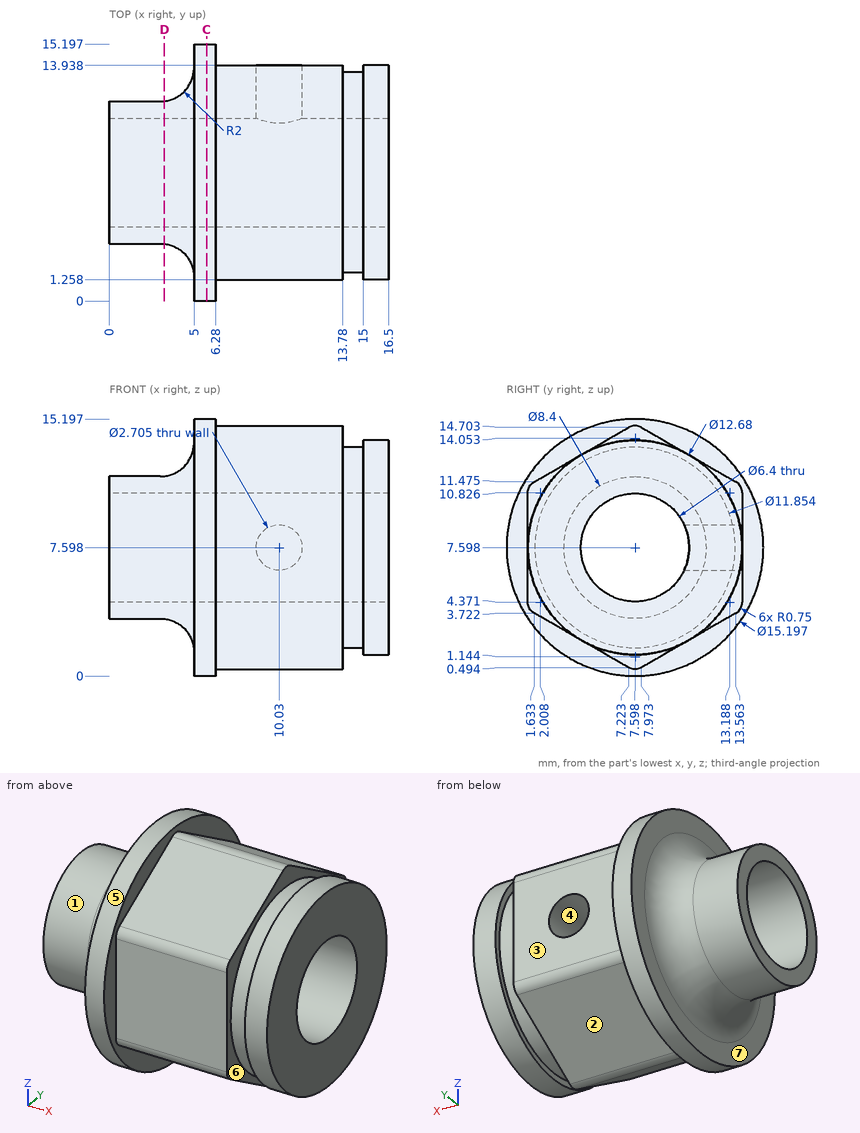
Job drawing, mm, ordinate dimensions from the low corner. One solid piece. A direction names the side the tool comes from. Give positions to 0.01 mm unless a question says otherwise; leave off trailing zeros. Loops run counter-clockwise (first coordinate to the right, second up) from the corner with the lowest first, then second, coordinate; pieces in that order, holes last. Notation, with made-up numbers: (5, -16.75) -> (52, -16.75) arc R29 cw to (52, 9.25) -> close; hole circle Ø7 at (-22, 38.5). An arc over 180 degrees is marked (long way). Write each question's results on one line, items separated by ' | '.
(1) Probe line 1 along Z through (x, y) = (7, 6.5) (1 decimal); line 2 along X through (y, z) = (1.75, 6) (1 decimal); line 3 along X through (y, z) = (12.5, 13). List the from-to ranges inside material, lowest first.
Geometry results:
line 1: z = 0.9 to 4.6, 10.6 to 14.3 | line 2: x = 5 to 13.8, 15 to 16.5 | line 3: x = 5 to 6.28
(2) Pull direction X, two halves, no side cores. Call the marked faces 5, 6 and 7: released by +X, released by -X, zero draft, split by the parting line, or undercut.
Geometry results:
face 5: zero draft | face 6: undercut | face 7: released by -X
(3) Cut at D-D on x = 3.25. List the corners of the cut face in (y, z) (1 decimal).
Geometry results:
outline: circle Ø8.4 at (7.6, 7.6); hole circle Ø6.4 at (7.6, 7.6)
(4) Flat gauge pins, fed straight in: pin 1 Ø1.5 at (y, z) = (8.5, 2) entering from -X; pin 2 Ø4 at (x, y) = (5.5, 1.5) entering from -Z; pin 3 Ø4 at (y, z) = (2, 13) entering from -X (1 decimal). Where does each tip first touch, or does it go through?
Geometry results:
pin 1: stops at x = 4.54 | pin 2: stops at z = 1.2 | pin 3: stops at x = 5
(5) Tool access for the marked faces 1, 2, 3 and 4: list every direction of +Z, -Z, +X, -X, +Y, -Y with a clear straight run to the whole face (end or side of a thin tool).
Geometry results:
face 1: -X | face 2: -Z, +X, +Y | face 3: +Z, -Z, +X, +Y | face 4: +Y
(6) Cut at C-C on x = 5.75. List the corners of the cut face in (y, z), and give its area (3 significant figures).
Geometry results:
outline: circle Ø15.2 at (7.6, 7.6); hole circle Ø6.4 at (7.6, 7.6) | area: 149 mm²
